Geometry: final body of the model. Coordinates: model frame, mm. Give positions to 0.01 mm unless a question says otherwise; leave off trailing zeros. Write each loop counter-clockwise with the first axis right and the second up, starting at its lowest first coordinate (ties: lowest second). Pieces come first, ordered by that corner, then holes. Notation, with made-up numbers: (78.25, 32.25) -> (92.25, 32.25) arc R26 ccw to (92.25, 68.25) -> close; hole circle Ø2 at (22, 5.25). An arc over 180 degrees is marked (long way). Answer as a JSON object with one key per item and string values.
from build123d import *

# Parameters (mm, degrees)
SKETCH1_W            = 240
SKETCH1_H            = 210
BOSS_EXTRUDE1_DEPTH  = 5
SKETCH2_W            = 240
SKETCH2_H            = 65
CUT_EXTRUDE1_DEPTH   = 5
SKETCH4_W            = 100
SKETCH4_H            = 5
BOSS_EXTRUDE2_DEPTH  = 10
SKETCH5_W            = 5
SKETCH5_H            = 35
SKETCH5_W_2          = 60
SKETCH5_H_2          = 5
CUT_EXTRUDE3_DEPTH   = 10
SKETCH6_W            = 5
SKETCH6_H            = 10
BOSS_EXTRUDE3_DEPTH  = 15
BOSS_EXTRUDE9_DEPTH  = 5
SKETCH13_W           = 5
SKETCH13_H           = 35
CUT_EXTRUDE4_DEPTH   = 10
SKETCH15_R           = 2.1
SKETCH15_W           = 15
SKETCH15_H           = 5.2
CUT_EXTRUDE8_DEPTH   = 10
SKETCH16_R           = 2.1
CUT_EXTRUDE9_DEPTH   = 10
SKETCH17_W           = 25
SKETCH17_H           = 5
SKETCH17_W_2         = 10
CUT_EXTRUDE10_DEPTH  = 10
SKETCH19_W           = 25
SKETCH19_H           = 5
SKETCH19_W_2         = 4
SKETCH19_H_2         = 3
SKETCH19_H_3         = 4
SKETCH19_W_3         = 1.5
CUT_EXTRUDE12_DEPTH  = 10
CUT_EXTRUDE13_DEPTH  = 10
SKETCH21_W           = 5
SKETCH21_H           = 25
CUT_EXTRUDE14_DEPTH  = 5
SKETCH22_W           = 5
SKETCH22_H           = 4.2
CUT_EXTRUDE15_DEPTH  = 5
SKETCH23_W           = 5
SKETCH23_H           = 25
CUT_EXTRUDE16_DEPTH  = 10
SKETCH24_W           = 5
SKETCH24_H           = 5
BOSS_EXTRUDE10_DEPTH = 5
SKETCH26_W           = 5
SKETCH26_H           = 5
BOSS_EXTRUDE12_DEPTH = 5
SKETCH27_R           = 2.5
CUT_EXTRUDE17_DEPTH  = 5
SKETCH28_W           = 5
SKETCH28_H           = 5
CUT_EXTRUDE18_DEPTH  = 10
SKETCH29_W           = 5
SKETCH29_H           = 5
CUT_EXTRUDE19_DEPTH  = 10
SKETCH30_W           = 10
SKETCH30_H           = 8.2
SKETCH30_W_2         = 4.2
SKETCH30_H_2         = 5
CUT_EXTRUDE20_DEPTH  = 10
SKETCH31_W           = 10
SKETCH31_H           = 5
CUT_EXTRUDE21_DEPTH  = 5
SKETCH32_W           = 20
SKETCH32_H           = 5
CUT_EXTRUDE22_DEPTH  = 5
SKETCH33_W           = 10
SKETCH33_H           = 1.8
CUT_EXTRUDE23_DEPTH  = 5
SKETCH34_R           = 2.1
SKETCH34_W           = 5
SKETCH34_H           = 10
CUT_EXTRUDE24_DEPTH  = 5


with BuildPart() as part:
    # Sketch1 → Boss-Extrude1 (new body)
    with BuildSketch(Plane.XY):
        with Locations((-120, 105)):
            Rectangle(SKETCH1_W, SKETCH1_H)
    extrude(amount=BOSS_EXTRUDE1_DEPTH)

    # Sketch2 → Cut-Extrude1 (cut)
    with BuildSketch(Plane.XY.offset(5)):
        with Locations((-120, 32.5)):
            Rectangle(SKETCH2_W, SKETCH2_H)
    extrude(amount=-CUT_EXTRUDE1_DEPTH, mode=Mode.SUBTRACT)

    # Sketch4 → Boss-Extrude2 (add)
    with BuildSketch(Plane.XZ.offset(-65)):
        with Locations((-170, 2.5)):
            Rectangle(SKETCH4_W, SKETCH4_H)
        with Locations((-70, 2.5)):
            Rectangle(SKETCH4_W, SKETCH4_H)
    extrude(amount=BOSS_EXTRUDE2_DEPTH)

    # Sketch5 → Cut-Extrude3 (cut)
    with BuildSketch(Plane.XY.offset(5)):
        with Locations((-237.5, 192.5)):
            Rectangle(SKETCH5_W, SKETCH5_H)
        with Locations((-2.5, 192.5)):
            Rectangle(SKETCH5_W, SKETCH5_H)
        with Locations((-50, 207.5)):
            Rectangle(SKETCH5_W_2, SKETCH5_H_2)
        with Locations((-190, 207.5)):
            Rectangle(SKETCH5_W_2, SKETCH5_H_2)
    extrude(amount=-CUT_EXTRUDE3_DEPTH, mode=Mode.SUBTRACT)

    # Sketch6 → Boss-Extrude3 (add)
    with BuildSketch(Plane.ZY.offset(220)):
        with Locations((2.5, 60)):
            Rectangle(SKETCH6_W, SKETCH6_H)
    boss_extrude3 = extrude(amount=BOSS_EXTRUDE3_DEPTH)

    # Mirror1: Boss-Extrude3 across plane
    add(boss_extrude3.mirror(Plane.ZY.offset(120)))

    # Sketch12 → Boss-Extrude9 (add)
    with BuildSketch(Plane.XY.offset(5)):
        with BuildLine():
            Line((-189.282032303, 55), (-50.717967697, 55))
            ThreePointArc((-50.717967697, 55), (-120, 15), (-189.282032303, 55))
        make_face()
    extrude(amount=-BOSS_EXTRUDE9_DEPTH)

    # Sketch13 → Cut-Extrude4 (cut)
    with BuildSketch(Plane.XY.offset(5)):
        with Locations((-237.5, 120)):
            Rectangle(SKETCH13_W, SKETCH13_H)
        with Locations((-2.5, 120)):
            Rectangle(SKETCH13_W, SKETCH13_H)
    extrude(amount=-CUT_EXTRUDE4_DEPTH, mode=Mode.SUBTRACT)

    # Sketch15 → Cut-Extrude8 (cut)
    with BuildSketch(Plane.XY):
        with Locations((-120, 177.5)):
            Circle(SKETCH15_R)
        with Locations((-142.5, 177.5)):
            Rectangle(SKETCH15_W, SKETCH15_H)
        with Locations((-97.5, 177.5)):
            Rectangle(SKETCH15_W, SKETCH15_H)
    extrude(amount=CUT_EXTRUDE8_DEPTH, mode=Mode.SUBTRACT)

    # Sketch16 → Cut-Extrude9 (cut)
    with BuildSketch(Plane.XY.offset(5)):
        Polygon((-160.98556701, 164.847268071), (-179.690721649, 147.960670133), (-183.041237113, 151.672010339), (-164.336082474, 168.558608278), align=None)
        Polygon((-201.810309278, 127.991597968), (-220.515463918, 111.10500003), (-223.865979381, 114.816340236), (-205.160824742, 131.702938175), align=None)
        with Locations((-192.425773196, 139.831804154)):
            Circle(SKETCH16_R)
        Polygon((-75.663917526, 168.558608278), (-56.958762887, 151.672010339), (-60.309278351, 147.960670133), (-79.01443299, 164.847268071), align=None)
        with Locations((-47.574226804, 139.831804154)):
            Circle(SKETCH16_R)
        Polygon((-34.839175258, 131.702938175), (-16.134020619, 114.816340236), (-19.484536082, 111.10500003), (-38.189690722, 127.991597968), align=None)
    extrude(amount=-CUT_EXTRUDE9_DEPTH, mode=Mode.SUBTRACT)

    # Sketch17 → Cut-Extrude10 (cut)
    with BuildSketch(Plane(origin=(0, 0, 0), x_dir=(-1, 0, 0), z_dir=(0, 0, -1))):
        with Locations((120, 57.5)):
            Rectangle(SKETCH17_W, SKETCH17_H)
        with Locations((152.5, 57.5)):
            Rectangle(SKETCH17_W_2, SKETCH17_H)
        with Locations((87.5, 57.5)):
            Rectangle(SKETCH17_W_2, SKETCH17_H)
    extrude(amount=-CUT_EXTRUDE10_DEPTH, mode=Mode.SUBTRACT)

    # Sketch19 → Cut-Extrude12 (cut)
    with BuildSketch(Plane(origin=(0, 0, 0), x_dir=(-1, 0, 0), z_dir=(0, 0, -1))):
        with Locations((120, 207.5)):
            Rectangle(SKETCH19_W, SKETCH19_H)
        with Locations((120, 202.5)):
            Rectangle(SKETCH19_W_2, SKETCH19_H)
        with Locations((120, 198.5)):
            Rectangle(SKETCH19_W_2, SKETCH19_H_2)
        with Locations((120, 195)):
            Rectangle(SKETCH19_W_2, SKETCH19_H_3)
        with Locations((122.75, 198.5)):
            Rectangle(SKETCH19_W_3, SKETCH19_H_2)
        with Locations((117.25, 198.5)):
            Rectangle(SKETCH19_W_3, SKETCH19_H_2)
    extrude(amount=-CUT_EXTRUDE12_DEPTH, mode=Mode.SUBTRACT)

    # Sketch20 → Cut-Extrude13 (cut)
    with BuildSketch(Plane.XY.offset(5)):
        Polygon((-273.079166664, 137.5), (-209.931771643, 137.5), (-173.918106282, 170.012336785), (-173.918106282, 219.696537232), (-273.079166664, 219.696537232), align=None)
        Polygon((33.079166664, 137.5), (33.079166664, 219.696537232), (-66.081893718, 219.696537232), (-66.081893718, 170.012336785), (-30.068228357, 137.5), align=None)
    extrude(amount=-CUT_EXTRUDE13_DEPTH, mode=Mode.SUBTRACT)

    # Sketch21 → Cut-Extrude14 (cut)
    with BuildSketch(Plane(origin=(0, 0, 0), x_dir=(0, 0, -1), z_dir=(1, 0, 0))):
        with Locations((-2.5, 77.5)):
            Rectangle(SKETCH21_W, SKETCH21_H)
    cut_extrude14 = extrude(amount=-CUT_EXTRUDE14_DEPTH, mode=Mode.SUBTRACT)

    # Mirror2: Cut-Extrude14 across plane
    add(cut_extrude14.mirror(Plane.ZY.offset(120)), mode=Mode.SUBTRACT)

    # Sketch22 → Cut-Extrude15 (cut)
    with BuildSketch(Plane.XY.offset(5)):
        with Locations((-7.5, 72.5)):
            Rectangle(SKETCH22_W, SKETCH22_H)
        with Locations((-7.5, 127.5)):
            Rectangle(SKETCH22_W, SKETCH22_H)
        Polygon((-10, 67.5), (-10, 70.4), (-10, 74.6), (-10, 77.5), (-16, 77.5), (-16, 67.5), align=None)
        Polygon((-10, 125.4), (-10, 129.6), (-10, 132.5), (-16, 132.5), (-16, 122.5), (-10, 122.5), align=None)
    cut_extrude15 = extrude(amount=-CUT_EXTRUDE15_DEPTH, mode=Mode.SUBTRACT)

    # Mirror3: Cut-Extrude15 across plane
    add(cut_extrude15.mirror(Plane(origin=(-120, 0, 0), x_dir=(0, 0, 1), z_dir=(1, 0, 0))), mode=Mode.SUBTRACT)

    # Sketch23 → Cut-Extrude16 (cut)
    with BuildSketch(Plane(origin=(0, 0, 0), x_dir=(-1, 0, 0), z_dir=(0, 0, -1))):
        with Locations((142.5, 112.5)):
            Rectangle(SKETCH23_W, SKETCH23_H)
        with Locations((97.5, 112.5)):
            Rectangle(SKETCH23_W, SKETCH23_H)
        with Locations((142.5, 177.5)):
            Rectangle(SKETCH23_W, SKETCH23_H)
        with Locations((97.5, 177.5)):
            Rectangle(SKETCH23_W, SKETCH23_H)
    extrude(amount=-CUT_EXTRUDE16_DEPTH, mode=Mode.SUBTRACT)

    # Sketch24 → Boss-Extrude10 (add)
    with BuildSketch(Plane.XY.offset(5)):
        with Locations((-97.5, 122.5)):
            Rectangle(SKETCH24_W, SKETCH24_H)
    extrude(amount=-BOSS_EXTRUDE10_DEPTH)

    # Sketch26 → Boss-Extrude12 (add)
    with BuildSketch(Plane.XY.offset(5)):
        with Locations((-142.5, 122.5)):
            Rectangle(SKETCH26_W, SKETCH26_H)
    extrude(amount=-BOSS_EXTRUDE12_DEPTH)

    # Sketch27 → Cut-Extrude17 (cut)
    with BuildSketch(Plane.XY.offset(5)):
        with Locations((-120, 105)):
            Circle(SKETCH27_R)
    extrude(amount=-CUT_EXTRUDE17_DEPTH, mode=Mode.SUBTRACT)

    # Sketch28 → Cut-Extrude18 (cut)
    with BuildSketch(Plane.ZY.offset(160)):
        with Locations((2.5, 207.5)):
            Rectangle(SKETCH28_W, SKETCH28_H)
    extrude(amount=-CUT_EXTRUDE18_DEPTH, mode=Mode.SUBTRACT)

    # Sketch29 → Cut-Extrude19 (cut)
    with BuildSketch(Plane(origin=(-80, 0, 0), x_dir=(0, 0, -1), z_dir=(1, 0, 0))):
        with Locations((-2.5, 207.5)):
            Rectangle(SKETCH29_W, SKETCH29_H)
    extrude(amount=-CUT_EXTRUDE19_DEPTH, mode=Mode.SUBTRACT)

    # Sketch30 → Cut-Extrude20 (cut)
    with BuildSketch(Plane.XY.offset(5)):
        with Locations((-77.5, 195.9)):
            Rectangle(SKETCH30_W, SKETCH30_H)
        with Locations((-77.5, 202.5)):
            Rectangle(SKETCH30_W_2, SKETCH30_H_2)
        Polygon((-157.5, 200), (-160.4, 200), (-164.6, 200), (-167.5, 200), (-167.5, 191.8), (-157.5, 191.8), align=None)
        with Locations((-162.5, 202.5)):
            Rectangle(SKETCH30_W_2, SKETCH30_H_2)
    extrude(amount=-CUT_EXTRUDE20_DEPTH, mode=Mode.SUBTRACT)

    # Sketch31 → Cut-Extrude21 (cut)
    with BuildSketch(Plane.XZ.offset(-55)):
        with Locations((-217.5, 2.5)):
            Rectangle(SKETCH31_W, SKETCH31_H)
        with Locations((-22.5, 2.5)):
            Rectangle(SKETCH31_W, SKETCH31_H)
    extrude(amount=-CUT_EXTRUDE21_DEPTH, mode=Mode.SUBTRACT)

    # Sketch32 → Cut-Extrude22 (cut)
    with BuildSketch(Plane.XY.offset(5)):
        with Locations((-139.918106282, 163.5)):
            Rectangle(SKETCH32_W, SKETCH32_H)
        with Locations((-99.918106282, 163.5)):
            Rectangle(SKETCH32_W, SKETCH32_H)
    extrude(amount=-CUT_EXTRUDE22_DEPTH, mode=Mode.SUBTRACT)

    # Sketch33 → Cut-Extrude23 (cut)
    with BuildSketch(Plane.XY.offset(5)):
        with Locations((-162.5, 190.9)):
            Rectangle(SKETCH33_W, SKETCH33_H)
        with Locations((-77.5, 190.9)):
            Rectangle(SKETCH33_W, SKETCH33_H)
    extrude(amount=-CUT_EXTRUDE23_DEPTH, mode=Mode.SUBTRACT)

    # Sketch34 → Cut-Extrude24 (cut)
    with BuildSketch(Plane.XY.offset(5)):
        with Locations((-218, 79)):
            Circle(SKETCH34_R)
        with Locations((-22, 79)):
            Circle(SKETCH34_R)
        with Locations((-218, 69)):
            Rectangle(SKETCH34_W, SKETCH34_H)
        with Locations((-218, 89)):
            Rectangle(SKETCH34_W, SKETCH34_H)
        with Locations((-22, 89)):
            Rectangle(SKETCH34_W, SKETCH34_H)
        with Locations((-22, 69)):
            Rectangle(SKETCH34_W, SKETCH34_H)
    extrude(amount=-CUT_EXTRUDE24_DEPTH, mode=Mode.SUBTRACT)


solid = part.part
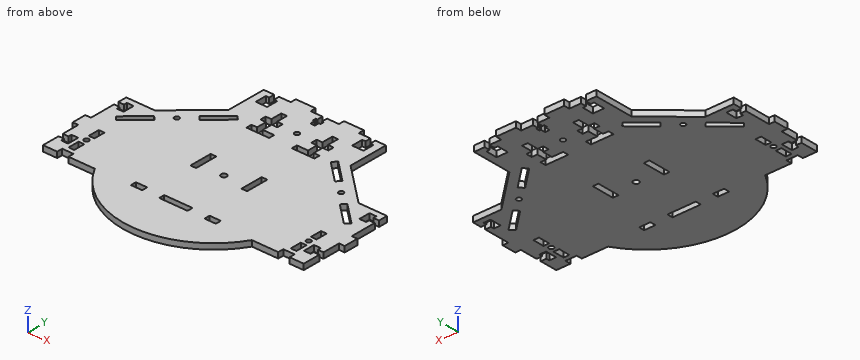
Q1. Cut plane A-A (y = 105). Return the cut outline in (x, z), and give its area (4 significant figures).
Values:
{"outline": "(-235, 0) -> (-145, 0) -> (-145, 5) -> (-235, 5) -> close; (-140, 0) -> (-122.5, 0) -> (-122.5, 5) -> (-140, 5) -> close; (-117.5, 0) -> (-100, 0) -> (-100, 5) -> (-117.5, 5) -> close; (-95, 0) -> (-5, 0) -> (-5, 5) -> (-95, 5) -> close", "area": "1,075 mm²"}
Q2. Cut plane B-B (y = 186). Return the cut outline in (x, z).
Values:
{"outline": "(-173.92, 0) -> (-145, 0) -> (-145, 5) -> (-173.92, 5) -> close; (-140, 0) -> (-100, 0) -> (-100, 5) -> (-140, 5) -> close; (-95, 0) -> (-66.08, 0) -> (-66.08, 5) -> (-95, 5) -> close"}
Q3. Material intervals for L1, parallel to Y at x = -119.5, z = 1.35; L2, parallel to X at y = 177.5, z = 4; L3, parallel to Y at x = -120, z = 3.45, sorted ascending. Write a range as from..to.
Values:
{"L1": "15..55, 60..102.55, 107.45..175.46, 179.54..193", "L2": "-173.92..-150, -135..-122.1, -117.9..-105, -90..-66.08", "L3": "15..55, 60..102.5, 107.5..175.4, 179.6..193"}
Q4. First-contact query: P1, Ø2.5, axis at y = 62.5, z = 2.5, coming from the -X side; P2, Ø1.5, axis at y = 208, z = 2.5, coming from the -X side; P3, Ø2.5, axis at x = -12, z = 2.5, coming from the +Y side. Flat tips, straight axial feed; report the tip coordinate or a pass-through.
Values:
{"P1": "x = -235", "P2": "x = -150", "P3": "y = 137.5"}
Q5. Cut plane C-C (z = 2.4). State how many separate pieces and enclosed holes the cut face has, and give its area (3 significant figures).
Values:
{"separate pieces": "1", "enclosed holes": "21", "area": "29,200 mm²"}
Q6. Cut plane D-D (y = 49). Return the cut outline in (x, z), and give its area (3 significant figures).
Values:
{"outline": "(-185.45, 0) -> (-54.55, 0) -> (-54.55, 5) -> (-185.45, 5) -> close", "area": "655 mm²"}
